The figure shows three views and two pictorial views of one solid part (mm, origin at its lowest corner). Answer the questions. A direction names the side the tool comes from. Coordinates: 2 decimals unless noted, no trailing zeros. Order: outer loops, then holes, each group sorted by start corner. A loop starts at its lowest first (then second) coordinate and runs counter-clockwise, first axis right, second up. Notation, with made-up numbers: M 48,-40 L 85,-40 A23 ccw 85,-12 Z; hole C 54,36.5 d9. An arc over 180 degrees is marked long. Write item = value, one per line. Start each with the question number.
Q1. Find section D-D on z = 5. Give the vertices of the cut face in (x, y) (3 decimals).
Q2. A tool of negligible diameter and unlimited length cuts with its end or side. For the marked faces 1 and 2, from which of +Z, -Z, +X, -X, +Y, -Y can it reach the whole face along a straight path? Write none if from no direction.
Q3. Determine the mould class of the marked faces 3, 4 and 5 for opening direction Y: released by +Y, released by -Y, zero draft, split by the parting line, or undercut.
Q4. This flat-tipped pin is pushed along its axis until it touches: P1, Ø6.5, axis at x = 9.525, y = 9.525, coming from the -Z side. Where does it stop, or does it pass through?
Q5. Find section B-B on z = 2.25. Give the vertices of the cut face in (x, y) (3 decimals).
Q6. Find section C-C on y = 10.25. Give the vertices of the cut face in (x, z) (3 decimals).
Q7. Straight lines are drawn through the part: line 1 along X through (y, z) = (19.5, 1) (3 decimals); line 2 along Z through (x, y) = (8.75, 15.25); line 3 along Y through (x, z) = (8.5, 3.75). For each, find the intervals that lie inside material, in ascending order.
Q8. Find section A-A on x = 7.5. Give the vertices of the cut face in (y, z), and give its area (3 significant figures).
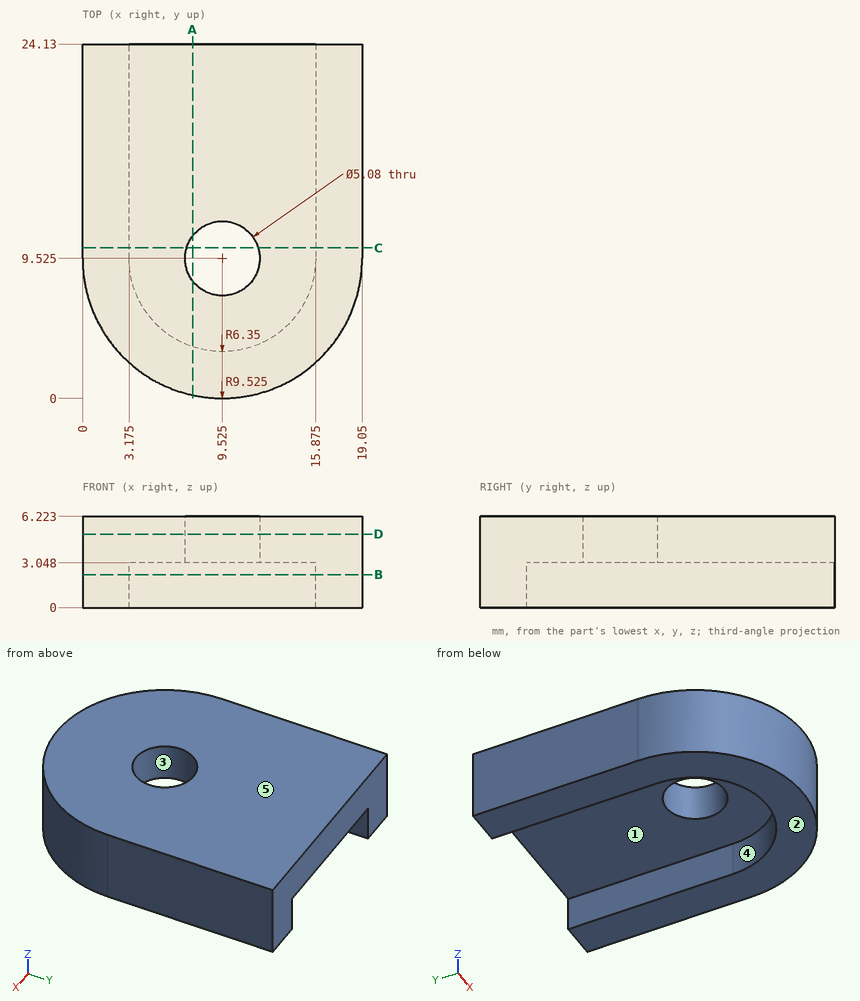
Findings below:
q1.outline = M 0,9.525 A9.525 ccw 19.05,9.525 L 19.05,24.13 L 0,24.13 Z; hole C 9.525,9.525 d5.08
q2.face_1 = -Z, +Y
q2.face_2 = -Z, +X, -X, +Y, -Y
q3.face_3 = undercut
q3.face_4 = released by +Y
q3.face_5 = zero draft
q4.P1 = 3.05
q5.outline = M 0,9.525 A9.525 ccw 19.05,9.525 L 19.05,24.13 L 15.875,24.13 L 15.875,9.525 A6.35 cw 3.175,9.525 L 3.175,24.13 L 0,24.13 Z
q6.outline = M 0,0 L 3.175,0 L 3.175,3.048 L 7.091,3.048 L 7.091,6.223 L 0,6.223 Z; M 11.959,3.048 L 15.875,3.048 L 15.875,0 L 19.05,0 L 19.05,6.223 L 11.959,6.223 Z
q7.line_1 = 0 to 3.175, 15.875 to 19.05
q7.line_2 = 3.05 to 6.22
q7.line_3 = 0.06 to 7.2, 11.85 to 24.13
q8.outline = M 0.22,0 L 3.51,0 L 3.51,3.05 L 7.99,3.05 L 7.99,6.22 L 0.22,6.22 Z; M 11.06,3.05 L 24.13,3.05 L 24.13,6.22 L 11.06,6.22 Z
q8.area = 76.2 mm^2
